Verification items for the finished model (mm, model axes). Face numbers are marked on the shaded views. A direction names the side the tool comes from. Round coordinates to 2 decimals unless told otherwise and drop trailing zeros. Loops run counter-clockwise (first coordinate to the right, second up) from the corner with the lowest first, then second, coordinate; pieces in that order, holes last. Notation, with made-up numbers: M 80,18 L 93,18 A11 cw 93,33 Z; hole C 13,86.5 d3. An arc over 180 degrees is marked long. One line per item, written item: value.
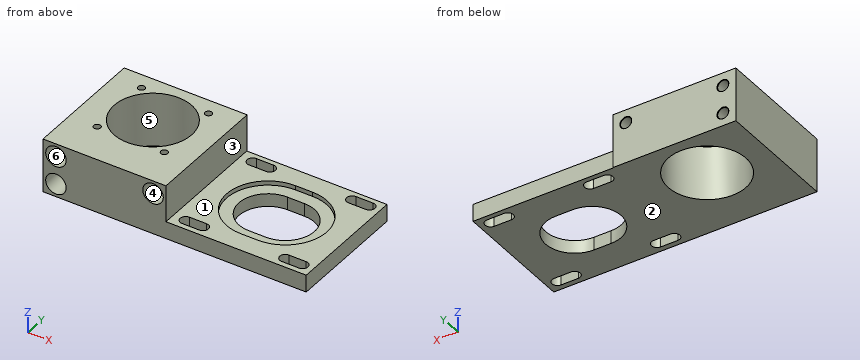
from build123d import *

# Parameters (mm, degrees)
F0_W     = 57
F0_H     = 57
F0_R     = 1.6
F0_R_2   = 18
F0_W_2   = 65
F1_DEPTH = 25
F2_DEPTH = 17
F3_DEPTH = 19
F4_R     = 2.55
F5_DEPTH = 60
F4_R_2   = 4.75
F6_DEPTH = 20
F7_DEPTH = 15
F8_W     = 65
F8_H     = 8
F9_DEPTH = 0.25
F10_SIZE = 0.2


# Not quite as in the source:
# - a feature names something its author has since deleted; it is built from what else it names


with BuildPart() as f1:
    # F0 (on Top) → F1 (new body)
    with BuildSketch(Plane.XY):
        with Locations((28.5, -28.5)):
            Rectangle(F0_W, F0_H)
        with Locations((12.9436508139, -38.5563491861)):
            Circle(F0_R, mode=Mode.SUBTRACT)
        with Locations((44.0563491861, -38.5563491861)):
            Circle(F0_R, mode=Mode.SUBTRACT)
        with Locations((28.5, -23)):
            Circle(F0_R_2, mode=Mode.SUBTRACT)
        with Locations((12.9436508139, -7.4436508139)):
            Circle(F0_R, mode=Mode.SUBTRACT)
        with Locations((44.0563491861, -7.4436508139)):
            Circle(F0_R, mode=Mode.SUBTRACT)
        with Locations((89.5, -28.5)):
            Rectangle(F0_W_2, F0_H)
        with BuildLine():
            Line((62.86, -49.45), (70.86, -49.45))
            ThreePointArc((70.86, -49.45), (73.41, -52), (70.86, -54.55))
            Line((70.86, -54.55), (62.86, -54.55))
            ThreePointArc((62.86, -54.55), (60.31, -52), (62.86, -49.45))
        make_face(mode=Mode.SUBTRACT)
        with BuildLine():
            Line((117, -54.55), (109, -54.55))
            ThreePointArc((109, -54.55), (106.45, -52), (109, -49.45))
            Line((109, -49.45), (117, -49.45))
            ThreePointArc((117, -49.45), (119.55, -52), (117, -54.55))
        make_face(mode=Mode.SUBTRACT)
        with BuildLine():
            Line((85.5, -9.25), (93.5, -9.25))
            ThreePointArc((93.5, -9.25), (112.75, -28.5), (93.5, -47.75))
            Line((93.5, -47.75), (85.5, -47.75))
            ThreePointArc((85.5, -47.75), (66.25, -28.5), (85.5, -9.25))
        make_face(mode=Mode.SUBTRACT)
        with BuildLine():
            Line((62.86, -2.45), (70.86, -2.45))
            ThreePointArc((70.86, -2.45), (73.41, -5), (70.86, -7.55))
            Line((70.86, -7.55), (62.86, -7.55))
            ThreePointArc((62.86, -7.55), (60.31, -5), (62.86, -2.45))
        make_face(mode=Mode.SUBTRACT)
        with BuildLine():
            Line((117, -7.55), (109, -7.55))
            ThreePointArc((109, -7.55), (106.45, -5), (109, -2.45))
            Line((109, -2.45), (117, -2.45))
            ThreePointArc((117, -2.45), (119.55, -5), (117, -7.55))
        make_face(mode=Mode.SUBTRACT)
        with Locations((12.9436508139, -7.4436508139)):
            Circle(F0_R)
        with Locations((44.0563491861, -7.4436508139)):
            Circle(F0_R)
        with Locations((44.0563491861, -38.5563491861)):
            Circle(F0_R)
        with Locations((12.9436508139, -38.5563491861)):
            Circle(F0_R)
        with BuildLine():
            ThreePointArc((93.5, -47.75), (112.75, -28.5), (93.5, -9.25))
            Line((93.5, -9.25), (85.5, -9.25))
            ThreePointArc((85.5, -9.25), (66.25, -28.5), (85.5, -47.75))
            Line((85.5, -47.75), (93.5, -47.75))
        make_face()
        with BuildLine():
            Line((85.5, -15), (93.5, -15))
            ThreePointArc((93.5, -15), (107, -28.5), (93.5, -42))
            Line((93.5, -42), (85.5, -42))
            ThreePointArc((85.5, -42), (72, -28.5), (85.5, -15))
        make_face(mode=Mode.SUBTRACT)
    extrude(amount=-F1_DEPTH)

    # F0 (on Top) → F2 (cut)
    with BuildSketch(Plane.XY):
        with Locations((89.5, -28.5)):
            Rectangle(F0_W_2, F0_H)
        with BuildLine():
            Line((62.86, -49.45), (70.86, -49.45))
            ThreePointArc((70.86, -49.45), (73.41, -52), (70.86, -54.55))
            Line((70.86, -54.55), (62.86, -54.55))
            ThreePointArc((62.86, -54.55), (60.31, -52), (62.86, -49.45))
        make_face(mode=Mode.SUBTRACT)
        with BuildLine():
            Line((117, -54.55), (109, -54.55))
            ThreePointArc((109, -54.55), (106.45, -52), (109, -49.45))
            Line((109, -49.45), (117, -49.45))
            ThreePointArc((117, -49.45), (119.55, -52), (117, -54.55))
        make_face(mode=Mode.SUBTRACT)
        with BuildLine():
            Line((85.5, -9.25), (93.5, -9.25))
            ThreePointArc((93.5, -9.25), (112.75, -28.5), (93.5, -47.75))
            Line((93.5, -47.75), (85.5, -47.75))
            ThreePointArc((85.5, -47.75), (66.25, -28.5), (85.5, -9.25))
        make_face(mode=Mode.SUBTRACT)
        with BuildLine():
            Line((62.86, -2.45), (70.86, -2.45))
            ThreePointArc((70.86, -2.45), (73.41, -5), (70.86, -7.55))
            Line((70.86, -7.55), (62.86, -7.55))
            ThreePointArc((62.86, -7.55), (60.31, -5), (62.86, -2.45))
        make_face(mode=Mode.SUBTRACT)
        with BuildLine():
            Line((117, -7.55), (109, -7.55))
            ThreePointArc((109, -7.55), (106.45, -5), (109, -2.45))
            Line((109, -2.45), (117, -2.45))
            ThreePointArc((117, -2.45), (119.55, -5), (117, -7.55))
        make_face(mode=Mode.SUBTRACT)
    extrude(amount=-F2_DEPTH, mode=Mode.SUBTRACT)

    # F0 (on Top) → F3 (cut)
    with BuildSketch(Plane.XY):
        with BuildLine():
            ThreePointArc((93.5, -47.75), (112.75, -28.5), (93.5, -9.25))
            Line((93.5, -9.25), (85.5, -9.25))
            ThreePointArc((85.5, -9.25), (66.25, -28.5), (85.5, -47.75))
            Line((85.5, -47.75), (93.5, -47.75))
        make_face()
        with BuildLine():
            Line((85.5, -15), (93.5, -15))
            ThreePointArc((93.5, -15), (107, -28.5), (93.5, -42))
            Line((93.5, -42), (85.5, -42))
            ThreePointArc((85.5, -42), (72, -28.5), (85.5, -15))
        make_face(mode=Mode.SUBTRACT)
        with BuildLine():
            ThreePointArc((93.5, -42), (107, -28.5), (93.5, -15))
            Line((93.5, -15), (85.5, -15))
            ThreePointArc((85.5, -15), (72, -28.5), (85.5, -42))
            Line((85.5, -42), (93.5, -42))
        make_face()
    extrude(amount=-F3_DEPTH, mode=Mode.SUBTRACT)

    # F4 (on face) → F5 (cut)
    with BuildSketch(Plane.XZ.offset(57)):
        with Locations((6, -6)):
            Circle(F4_R)
        with Locations((6, -19)):
            Circle(F4_R)
        with Locations((51, -6)):
            Circle(F4_R)
    extrude(amount=-F5_DEPTH, mode=Mode.SUBTRACT)

    # F4 (on face) → F6 (cut)
    with BuildSketch(Plane.XZ.offset(57)):
        with Locations((6, -6)):
            Circle(F4_R_2)
        with Locations((6, -6)):
            Circle(F4_R, mode=Mode.SUBTRACT)
        with Locations((6, -19)):
            Circle(F4_R_2)
        with Locations((6, -19)):
            Circle(F4_R, mode=Mode.SUBTRACT)
        with Locations((51, -6)):
            Circle(F4_R_2)
        with Locations((51, -6)):
            Circle(F4_R, mode=Mode.SUBTRACT)
    extrude(amount=-F6_DEPTH, mode=Mode.SUBTRACT)

    # F0 (on Top) → F7 (cut)
    with BuildSketch(Plane.XY):
        with Locations((44.0563491861, -7.4436508139)):
            Circle(F0_R)
        with Locations((44.0563491861, -38.5563491861)):
            Circle(F0_R)
        with Locations((12.9436508139, -38.5563491861)):
            Circle(F0_R)
        with Locations((12.9436508139, -7.4436508139)):
            Circle(F0_R)
    extrude(amount=-F7_DEPTH, mode=Mode.SUBTRACT)

    # F8 (on face) → F9 (cut)
    with BuildSketch(Plane(origin=(0, 0, 0), x_dir=(-1, 0, 0), z_dir=(0, 1, 0))):
        with Locations((-89.5, -21)):
            Rectangle(F8_W, F8_H)
    extrude(amount=-F9_DEPTH, mode=Mode.SUBTRACT)

    # F10
    f10_edges = [f1.edges().sort_by_distance(p)[0] for p in [
        (48.45, 0, -6),
        (3.45, 0, -6),
        (3.45, 0, -19),
    ]]
    chamfer(f10_edges, length=F10_SIZE)


solid = f1.part
(1) Sectioned sample at A-A on x = 51. Enter the section's corners in (y, z).
Completed:
outline: M -57,-25 L 0,-25 L 0,-8.75 L -0.2,-8.55 L -37,-8.55 L -37,-10.75 L -57,-10.75 Z; M -57,-1.25 L -37,-1.25 L -37,-3.45 L -0.2,-3.45 L 0,-3.25 L 0,0 L -57,0 Z
(2) Sectioned sample at C-C on y = -24.5. Enter the section's corners in (x, z), and give its area (3 significant figures).
Completed:
outline: M 0,-25 L 10.56,-25 L 10.56,0 L 0,0 Z; M 46.44,-25 L 72.61,-25 L 72.61,-19 L 66.67,-19 L 66.67,-17 L 57,-17 L 57,0 L 46.44,0 Z; M 106.39,-25 L 122,-25 L 122,-17 L 112.33,-17 L 112.33,-19 L 106.39,-19 Z; hole C 6,-19 d5.1; hole C 6,-6 d5.1; hole C 51,-6 d5.1
area: 693 mm^2
(3) Mould release check, pull along Z, two halves, no side actions. Record for the marked faces 1, 2, 3 and 4: +Z half, -Z half, draft (parallel to the pull), parting line (faces both ways), or undercut.
Completed:
face 1: +Z half
face 2: -Z half
face 3: draft
face 4: undercut
(4) Thickness scan on L1, parallel to Z at x = 6, y = -49; L2, parallel to Z at x = 6, y = -22; L3, parallel to X at y = -30, z = -6.25. Record the ranges inside material, lowest first. Write a range as from..to.
Completed:
L1: z = -25..-23.75, -14.25..-10.75, -1.25..0
L2: z = -25..-21.55, -16.45..-8.55, -3.45..0
L3: x = 0..3.46, 8.54..11.92, 45.08..48.46, 53.54..57
(5) Tool access check on the marked faces 5 and 6. Record the directions out of +Z, -Z, +X, -X, +Y, -Y that give a thin tool (end or side, any length) a straight path to the whole face; none if there is none.
Completed:
face 5: +Z, -Z
face 6: -Y
(6) Sectioned sample at D-D on x = 90.5. Enter the section's corners in (y, z), and give its area (3 significant figures).
Completed:
outline: M -57,-25 L -42,-25 L -42,-19 L -47.75,-19 L -47.75,-17 L -57,-17 Z; M -15,-25 L -0.25,-25 L -0.25,-17 L -9.25,-17 L -9.25,-19 L -15,-19 Z
area: 215 mm^2
(7) Sectioned sample at B-B on z = -6. Count the separate pieces of the cut face and the enclosed holes in it, and give its area (3 significant figures).
Completed:
separate pieces: 3
enclosed holes: 5
area: 1,440 mm^2
(8) Depth check by flat-ended pin: pin 1 Ø3 at (x, z) = (51, -6) entering from -Y; pin 2 Ø8 at (y, z) = (-12, -5.5) entering from -X; pin 3 Ø2.5 at (x, z) = (113, -20) entering from +Y; pin 4 Ø7.5 at (y, z) = (-18.5, -11.5) entering from +X. Enter the tip coordinate at first touch or a pass-through.
Completed:
pin 1: passes through
pin 2: stops at x = 0
pin 3: stops at y = -0.25
pin 4: stops at x = 57
